```python
from build123d import *

# Parameters (mm, degrees)
SKETCH1_W                 = 25
SKETCH1_H                 = 55
BOSS_EXTRUDE1_DEPTH       = 3
F_8_0MM_DOWEL_HOLE1_D     = 8
F_8_0MM_DOWEL_HOLE1_DEPTH = 3
F_8_0MM_DOWEL_HOLE1_TIP   = 2.403442476
F_3_0MM_DOWEL_HOLE1_D     = 3
F_3_0MM_DOWEL_HOLE1_DEPTH = 3
F_3_0MM_DOWEL_HOLE1_TIP   = 0.901290929
SKETCH6_W                 = 25
SKETCH6_H                 = 3
BOSS_EXTRUDE2_DEPTH       = 67
CUT_EXTRUDE2_DEPTH        = 90.895772982
F_8_0MM_DOWEL_HOLE2_D     = 8
F_3_0MM_DOWEL_HOLE2_D     = 3
FILLET2_R                 = 0.5


with BuildPart() as part:
    # Sketch1 → Boss-Extrude1 (new body)
    with BuildSketch(Plane.XY):
        Rectangle(SKETCH1_W, SKETCH1_H)
    extrude(amount=BOSS_EXTRUDE1_DEPTH)

    # Ø8.0mm Dowel Hole1
    with Locations(Plane.XY.offset(3)):
        with Locations((0, 0)):
            Hole(F_8_0MM_DOWEL_HOLE1_D / 2, depth=F_8_0MM_DOWEL_HOLE1_DEPTH)
            with Locations((0, 0, -(F_8_0MM_DOWEL_HOLE1_DEPTH + F_8_0MM_DOWEL_HOLE1_TIP / 2))):  # 118° drill point
                Cone(0, F_8_0MM_DOWEL_HOLE1_D / 2, F_8_0MM_DOWEL_HOLE1_TIP, mode=Mode.SUBTRACT)

    # Ø3.0mm Dowel Hole1
    with Locations(Plane.XY.offset(3)):
        with Locations((0, -7.946297912), (-7.946297912, 0), (0, 7.946297912), (7.946297912, 0), (0, 0), (0, 18), (0, -36), (0, -18)):
            Hole(F_3_0MM_DOWEL_HOLE1_D / 2, depth=F_3_0MM_DOWEL_HOLE1_DEPTH)
            with Locations((0, 0, -(F_3_0MM_DOWEL_HOLE1_DEPTH + F_3_0MM_DOWEL_HOLE1_TIP / 2))):  # 118° drill point
                Cone(0, F_3_0MM_DOWEL_HOLE1_D / 2, F_3_0MM_DOWEL_HOLE1_TIP, mode=Mode.SUBTRACT)

    # Sketch6 → Boss-Extrude2 (add)
    with BuildSketch(Plane.XY.offset(3)):
        with Locations((0, 26)):
            Rectangle(SKETCH6_W, SKETCH6_H)
        with Locations((0, -26)):
            Rectangle(SKETCH6_W, SKETCH6_H)
    extrude(amount=BOSS_EXTRUDE2_DEPTH)

    # Sketch8 → Cut-Extrude2 (cut, through all)
    with BuildSketch(Plane(origin=(0, 27.5, 0), x_dir=(1, 0, 0), z_dir=(0, 1, 0))):
        with BuildLine():
            Line((-12.5, -57.5), (-12.5, -70))
            Line((-12.5, -70), (0, -70))
            ThreePointArc((0, -70), (-8.838834765, -66.338834765), (-12.5, -57.5))
        make_face()
        with BuildLine():
            ThreePointArc((12.5, -57.5), (8.838834765, -66.338834765), (0, -70))
            Line((0, -70), (12.5, -70))
            Line((12.5, -70), (12.5, -57.5))
        make_face()
    extrude(amount=-CUT_EXTRUDE2_DEPTH, mode=Mode.SUBTRACT)

    # Ø8.0mm Dowel Hole2 (through all)
    with Locations(Plane(origin=(0, 27.5, 0), x_dir=(1, 0, 0), z_dir=(0, 1, 0))):
        with Locations((0, -57.5)):
            Hole(F_8_0MM_DOWEL_HOLE2_D / 2)

    # Ø3.0mm Dowel Hole2 (through all)
    with Locations(Plane(origin=(0, 27.5, 0), x_dir=(1, 0, 0), z_dir=(0, 1, 0))):
        with Locations((0, -57.5), (0.326210902, -39.5), (-0.326210902, -21.5), (0, -50.5), (7, -57.5), (0, -64.5), (-7, -57.5)):
            Hole(F_3_0MM_DOWEL_HOLE2_D / 2)

    # Fillet2
    fillet2_edges = [part.edges().sort_by_distance(p)[0] for p in [
        (12.5, 27.5, 28.75),
        (12.5, 24.5, 30.25),
        (12.5, -24.5, 30.25),
        (12.5, -27.5, 28.75),
        (0, -27.5, 0),
        (-12.5, 0, 0),
        (0, 27.5, 0),
        (-12.5, 0, 3),
        (12.5, 0, 0),
        (12.5, 0, 3),
        (-12.5, -24.5, 30.25),
        (-12.5, 24.5, 30.25),
        (-12.5, -27.5, 28.75),
        (-12.5, 27.5, 28.75),
        (0, 27.5, 70),
        (0, 24.5, 70),
        (0, -24.5, 70),
        (0, -27.5, 70),
    ]]
    fillet(fillet2_edges, radius=FILLET2_R)


solid = part.part
```
Check sheet for the modelled part. Datum: model origin and axes. Units: mm. Round coordinates to 2 decimals unless told otherwise and drop trailing zeros. Loops run counter-clockwise (first coordinate to the right, second up) from the corner with the lowest first, then second, coordinate; pieces in that order, holes last. Notation, with made-up numbers: M 69.25,57.5 L 85.25,57.5 A12 ccw 85.25,72.5 Z; hole C 29.25,86.5 d7. An arc over 180 degrees is marked long. Answer as a JSON object with one key per item and string values.
1. Section check A-A (z = 50.5). Record the boundary of the cut face in (x, y).
Reply:
{"outline": "M -12.5,-27 A0.5 ccw -12,-27.5 L -1.5,-27.5 L -1.5,-24.5 L -12,-24.5 A0.5 ccw -12.5,-25 Z; M -12.5,25 A0.5 ccw -12,24.5 L -1.5,24.5 L -1.5,27.5 L -12,27.5 A0.5 ccw -12.5,27 Z; M 1.5,-27.5 L 12,-27.5 A0.5 ccw 12.5,-27 L 12.5,-25 A0.5 ccw 12,-24.5 L 1.5,-24.5 Z; M 1.5,24.5 L 12,24.5 A0.5 ccw 12.5,25 L 12.5,27 A0.5 ccw 12,27.5 L 1.5,27.5 Z"}
2. Section check C-C (z = 19). Record the boundary of the cut face in (x, y).
Reply:
{"outline": "M -12.5,-27 A0.5 ccw -12,-27.5 L 12,-27.5 A0.5 ccw 12.5,-27 L 12.5,-25 A0.5 ccw 12,-24.5 L -12,-24.5 A0.5 ccw -12.5,-25 Z; M -12.5,25 A0.5 ccw -12,24.5 L 12,24.5 A0.5 ccw 12.5,25 L 12.5,27 A0.5 ccw 12,27.5 L -12,27.5 A0.5 ccw -12.5,27 Z"}
3. Section check D-D (y = -10.5). Record the boundary of the cut face in (x, z), plus the area to 3 significant figures.
Reply:
{"outline": "M -12.5,0.5 A0.5 ccw -12,0 L 12,0 A0.5 ccw 12.5,0.5 L 12.5,2.5 A0.5 ccw 12,3 L -12,3 A0.5 ccw -12.5,2.5 Z", "area": "74.8 mm²"}
4. Mould release check, pull along Y, two halves, no side actions. Record for faces 1 (the flat face through (0, -24.5, 36)), 2 (the flat face through (0, -27.5, 35)), 3 (the cylindrical face through (7, -26, 56)): pulls with the +Y half, pulls with the -Y half, needs draft (parallel to the pull), parting line crosses it, or undercut.
Reply:
{"face 1": "undercut", "face 2": "pulls with the -Y half", "face 3": "needs draft"}
5. Section check B-B (y = -18). Record the boundary of the cut face in (x, z), plus the area to 3 significant figures.
Reply:
{"outline": "M -12.5,0.5 A0.5 ccw -12,0 L -1.5,0 L -1.5,3 L -12,3 A0.5 ccw -12.5,2.5 Z; M 1.5,0 L 12,0 A0.5 ccw 12.5,0.5 L 12.5,2.5 A0.5 ccw 12,3 L 1.5,3 Z", "area": "65.8 mm²"}
6. Gauge pin test, flat end, axial feed: P1, Ø5, axis at x = 7.95, y = 0, coming from the +Z side. Record the tip position at first contact, or that the pin passes through.
Reply:
{"P1": "stops at z = 3"}
7. Scan lines: line 1 (X direction, y = 0, z = 2); line 2 (Y direction, x = 0, z = 2.3); line 3 (Y direction, x = -8.75, z = 25). Record each from-to range of solid material in increasing order.
Reply:
{"line 1": "x = -12.5 to -9.45, -6.45 to -4, 4 to 6.45, 9.45 to 12.5", "line 2": "y = -27.5 to -19.5, -16.5 to -9.45, -6.45 to -4, 4 to 6.45, 9.45 to 16.5, 19.5 to 27.5", "line 3": "y = -27.5 to -24.5, 24.5 to 27.5"}
